Could you check a few things on this model? Use its own coordinates, in mm. Face numbers are marked on the shaded views. Coordinates: 2 decimals unless noted, no trailing zeros. Write each loop counter-clockwise with the first axis right and the second up, starting at its lowest first coordinate (ties: lowest second). Pieces come first, ordered by that corner, then holes. Notation, with made-up numbers: M 47,46 L 72,46 A35 ccw 72,80 Z; hole C 6,67.5 d10. An arc over 180 degrees is marked long. Write item = value, one per line.
```python
from build123d import *

# Parameters (mm, degrees)
SKETCH1_R           = 9.15
SKETCH1_R_2         = 7.65
BOSS_EXTRUDE1_DEPTH = 40
SKETCH2_W           = 6
SKETCH2_H           = 6
CUT_EXTRUDE1_DEPTH  = 15
SKETCH3_W           = 2
SKETCH3_H           = 3
CHAMFER1_SIZE       = 2
CUT_EXTRUDE2_DEPTH  = 5


with BuildPart() as part:
    # Sketch1 → Boss-Extrude1 (new body)
    with BuildSketch(Plane.XY):
        Circle(SKETCH1_R)
        Circle(SKETCH1_R_2, mode=Mode.SUBTRACT)
    extrude(amount=BOSS_EXTRUDE1_DEPTH)

    # Sketch2 → Cut-Extrude1 (cut, symmetric)
    with BuildSketch(Plane(origin=(0, 0, 0), x_dir=(1, 0, 0), z_dir=(0, 1, 0))):
        with Locations((0, -37)):
            Rectangle(SKETCH2_W, SKETCH2_H)
    extrude(amount=CUT_EXTRUDE1_DEPTH, both=True, mode=Mode.SUBTRACT)

    # Sketch3 → Revolve1 (revolve)
    with BuildSketch(Plane(origin=(0, 0, 0), x_dir=(1, 0, 0), z_dir=(0, 1, 0)), mode=Mode.PRIVATE) as revolve1_sk:
        with Locations((10.15, -29.5)):
            Rectangle(SKETCH3_W, SKETCH3_H)
        with Locations((10.15, -1.5)):
            Rectangle(SKETCH3_W, SKETCH3_H)
    revolve(revolve1_sk.sketch.rotate(Axis((0, 0, 0), (0, 0, 1)), 180), axis=Axis((0, 0, 0), (0, 0, 1)))

    # Chamfer1
    chamfer1_edges = [part.edges().sort_by_distance(p)[0] for p in [
        (11.15, 0, 28),
        (11.15, 0, 3),
    ]]
    chamfer(chamfer1_edges, length=CHAMFER1_SIZE - 0.0001)  # a hair under: the kernel refuses the full size

    # Sketch4 → Cut-Extrude2 (cut)
    with BuildSketch(Plane(origin=(0, 0, 0), x_dir=(-1, 0, 0), z_dir=(0, 0, -1))):
        with BuildLine():
            Line((0.5, -9.136328584), (0.609289617, -11.133340297))
            ThreePointArc((0.609289617, -11.133340297), (0, -11.15), (-0.609289617, -11.133340297))
            Line((-0.609289617, -11.133340297), (-0.5, -9.136328584))
            ThreePointArc((-0.5, -9.136328584), (0, -9.15), (0.5, -9.136328584))
        make_face()
    extrude(amount=-CUT_EXTRUDE2_DEPTH, mode=Mode.SUBTRACT)


solid = part.part
```
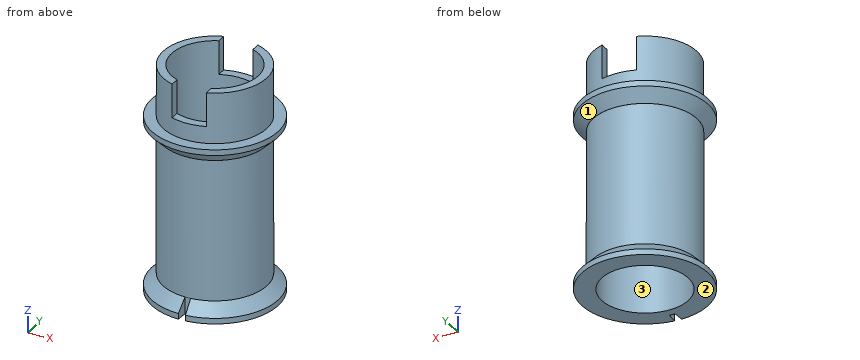
Item 1: Imagine slicing it at C-C (z = 30.5). Write out the boundary of the cut face in (x, y), and give its area (3 significant figures).
Numbers:
outline = C 0,0 d22.3; hole C 0,0 d15.3
area = 207 mm²
Item 2: I'm going to push flat-ended pins straight in: P1, Ø0.8, axis at y = -8, z = 35.5, coming from the +X side; P2, Ø5, axis at y = -4.5, z = 17, coming from the -X side; P3, Ø0.6, axis at x = 0, y = -8, coming from the +Z side. Where does each tip first touch, or does it pass through?
Numbers:
P1 = 5.1
P2 = -8.93
P3 = 34
Item 3: If we mould it in two halves opening along Z, with no side actions, what happens to the marked faces 1, 2 and 3? For each: pulls with the +Z half, pulls with the -Z half, needs draft (parallel to the pull), parting line crosses it, or undercut.
Numbers:
face_1 = undercut
face_2 = pulls with the -Z half
face_3 = needs draft
Item 4: Imagine slicing it at B-B (z = 11.5). Write out the boundary of the cut face in (x, y), and give its area (3 significant figures).
Numbers:
outline = C 0,0 d18.3; hole C 0,0 d15.3
area = 79.2 mm²
Item 5: If I drill on line 1 along Y through (x, z) = (0, 20.5); line 2 along X through (y, z) = (-5, 38); line 3 along Z through (x, y) = (-9.25, 2.75), over which ranges is the centre line in solid material (lowest first)?
Numbers:
line_1 = -9.15 to -7.65, 7.65 to 9.15
line_2 = -7.66 to -5.79, 5.79 to 7.66
line_3 = 0 to 2.5, 28.5 to 31
Item 6: Imagine slicing it at A-A (z = 36). Write out the boundary of the cut face in (x, y), and give its area (3 significant figures).
Numbers:
outline = M -3,-8.64 L -3,-7.04 A7.65 cw -3,7.04 L -3,8.64 A9.15 ccw Z; M 3,-8.64 A9.15 ccw 3,8.64 L 3,7.04 A7.65 cw 3,-7.04 Z
area = 60.8 mm²
